Source: CAD feature listing. Evaluate the final solid. Frame: model axes, mm. Give positions to 0.01 mm unless a question says otherwise; leave off trailing zeros. Order: outer loops, then holes, each group sorted by start corner. A loop starts at its lowest first (then second) coordinate and runs counter-clockwise, first axis right, second up. Notation, with made-up numbers: M -28,64 L 18,64 A18 cw 18,70 Z; hole C -39,-5 d10. An arc over 180 degrees is marked long. Answer in a Markdown table with one row per item. Add a question column.
(1) Mould query, pull axis Y, two halves, no side actions, for faces 1 (the face through (1.61, -16.43, 0.26)), 2 (the face through (2, -1, 42.5)), 3 (the face through (1.61, -42.649, 41.776)). Classes: pulls with the +Y half, pulls with the -Y half, needs draft (parallel to the pull), parting line crosses it, or undercut.
(2) Section query A-A, the plane z = 0. Return loops of the section in (x, y) (1 decimal), plus the area to 3 significant figures.
(3) Pin query (flat end, axial travel): P1, Ø3, axis at y = -18.41, z = 0, coming from the -X side. Return the tip coordinate at first contact, or that it passes through.
(4) Material intervals for line 1 along Y through (x, z) = (1.85, 0); line 2 along Z through (x, y) = (2.25, -20); line 3 along Z through (x, y) = (1.8, -19.5), sorted ascending.
from build123d import *

# Parameters (mm, degrees)
SKETCH1_W           = 84.999999926
SKETCH1_H           = 86.825000086
BOSS_EXTRUDE1_DEPTH = 3.175
SKETCH2_R           = 2
CUT_EXTRUDE1_DEPTH  = 61.835645652
FILLET1_R           = 2.54


with BuildPart() as part:
    # Sketch1 → Boss-Extrude1 (new body)
    with BuildSketch(Plane(origin=(0, 0, 0), x_dir=(0, 0, -1), z_dir=(1, 0, 0))):
        Rectangle(SKETCH1_W, SKETCH1_H)
    extrude(amount=BOSS_EXTRUDE1_DEPTH)

    # Sketch2 → Cut-Extrude1 (cut, through all)
    with BuildSketch(Plane(origin=(3.175, 0, 0), x_dir=(0, 0, -1), z_dir=(1, 0, 0))):
        with Locations((3.7e-08, -18.412500043)):
            Circle(SKETCH2_R)
    extrude(amount=-CUT_EXTRUDE1_DEPTH, mode=Mode.SUBTRACT)

    # Fillet1
    fillet1_edges = [part.edges().sort_by_distance(p)[0] for p in [
        (1.5875, 43.412500043, 42.499999963),
        (1.5875, 43.412500043, -42.499999963),
        (1.5875, -43.412500043, -42.499999963),
        (1.5875, -43.412500043, 42.499999963),
    ]]
    fillet(fillet1_edges, radius=FILLET1_R)


solid = part.part
Values follow:
| question | item | result |
|---|---|---|
| 1 | face 1 | undercut |
| 1 | face 2 | needs draft |
| 1 | face 3 | pulls with the -Y half |
| 2 | outline | M 0,-43.4 L 3.2,-43.4 L 3.2,-20.4 L 0,-20.4 Z; M 0,-16.4 L 3.2,-16.4 L 3.2,43.4 L 0,43.4 Z |
| 2 | area | 263 mm² |
| 3 | P1 | passes through |
| 4 | line 1 | y = -43.41 to -20.41, -16.41 to 43.41 |
| 4 | line 2 | z = -42.5 to -1.22, 1.22 to 42.5 |
| 4 | line 3 | z = -42.5 to -1.68, 1.68 to 42.5 |
